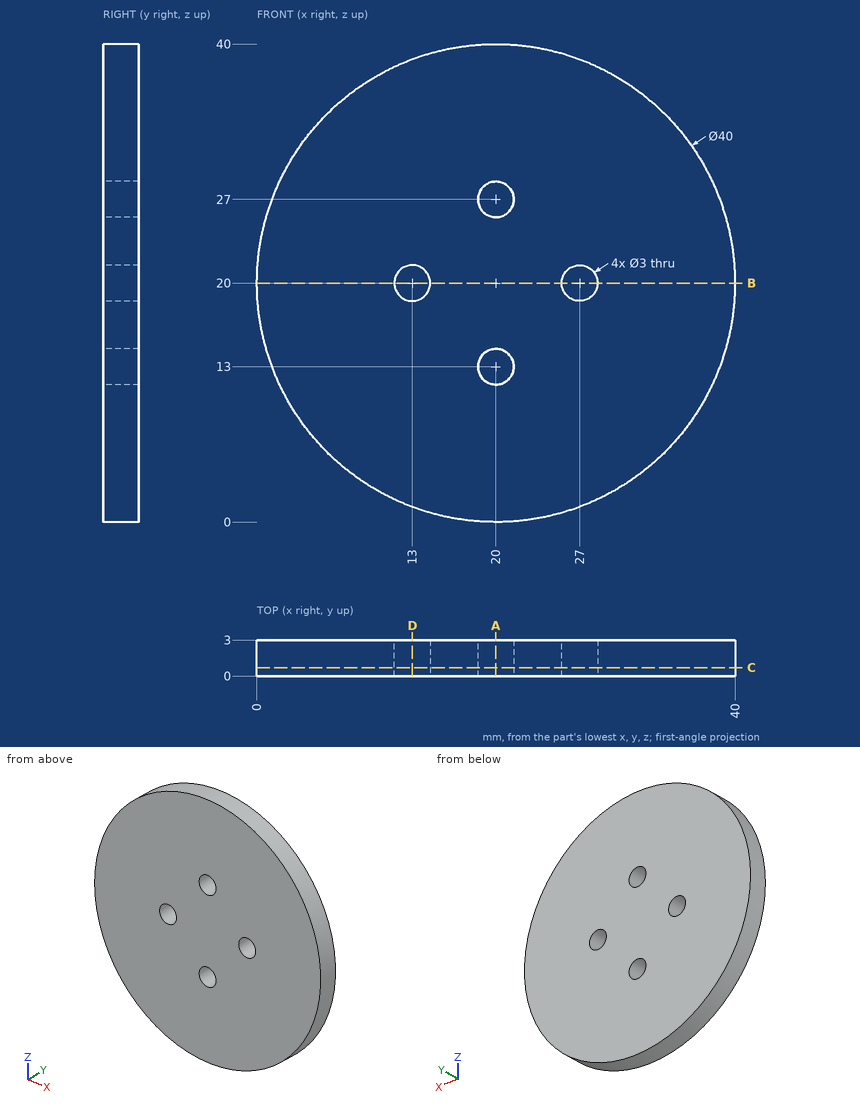
Geometry: see drawing. Coordinates: mm, zero at the bounding-box minimum. Coordinates: 2 decimals unless noted, no trailing zeros. Loops run counter-clockwise (first coordinate to the right, second up) from the corner with the lowest first, then second, coordinate; pieces in that order, holes last.
Q1. Cut plane C-C (y = 0.7). Output: boundary loops of the cut face in (x, z), then the cut area to 3 significant figures.
Q2. Cut plane D-D (x = 13). Output: boundary loops of the cut face in (y, z) (3 decimals), then the cut area to 3 significant figures.
Q3. Material intervals for line 1 (Z direction, x = 20, y = 1.95); line 2 (Z direction, x = 19, y = 0.3), sorted ascending.
Q4. Cut plane A-A (x = 20). Output: boundary loops of the cut face in (y, z).
Q5. Cut plane B-B (z = 20). Output: boundary loops of the cut face in (x, y).
Q6. Contact query for flat-ended pins moving along their axis: pin 1 (1 mm diameter, centred on x = 34.5, y = 1, fed in from +Z); pin 2 (1.8 mm diameter, centred on x = 27, z = 20, fed in from -Y); pin 3 (1 mm diameter, centred on y = 1, z = 11.5, fed in from +X); pin 4 (3.5 mm diameter, centred on x = 13, z = 20, fed in from +Y). Output: stop coordinate, or through.
Working result:
1. outline: circle Ø40 at (20, 20); hole circle Ø3 at (13, 20); hole circle Ø3 at (20, 13); hole circle Ø3 at (20, 27); hole circle Ø3 at (27, 20)
1. area: 1,230 mm2
2. outline: (0, 1.265) - (3, 1.265) - (3, 18.5) - (0, 18.5) - close; (0, 21.5) - (3, 21.5) - (3, 38.735) - (0, 38.735) - close
2. area: 103 mm2
3. line 1: z = 0 to 11.5, 14.5 to 25.5, 28.5 to 40
3. line 2: z = 0.03 to 11.88, 14.12 to 25.88, 28.12 to 39.97
4. outline: (0, 0) - (3, 0) - (3, 11.5) - (0, 11.5) - close; (0, 14.5) - (3, 14.5) - (3, 25.5) - (0, 25.5) - close; (0, 28.5) - (3, 28.5) - (3, 40) - (0, 40) - close
5. outline: (0, 0) - (11.5, 0) - (11.5, 3) - (0, 3) - close; (14.5, 0) - (25.5, 0) - (25.5, 3) - (14.5, 3) - close; (28.5, 0) - (40, 0) - (40, 3) - (28.5, 3) - close
6. pin 1: stops at z = 34.28
6. pin 2: passes through
6. pin 3: stops at x = 38.33
6. pin 4: stops at y = 3
